Verification items for the finished model (mm, model axes). A direction names the side the tool comes from. Give positions to 0.01 mm unless a question says otherwise; leave off trailing zeros. Loops run counter-clockwise (first coordinate to the right, second up) from the corner with the lowest first, then second, coordinate; pieces in that order, holes last. Notation, with made-up numbers: (18.25, -14.75) - (77.25, -14.75) arc R20 cw to (77.25, 16.25) - close; hole circle Ø3 at (-12, 40). An arc over 180 degrees is marked (long way). One line per question, with ' | ' between items. Start each with the question number.
1. Section check B-B, the plane x = 12. Enter the section's corners in (y, z).
2. Section check A-A, the plane y = 19. Enter the section's corners in (x, z).
3. Tool access check on faces 1 (the face through (27, 69.85, -3)), 2 (the face through (22.86, 16, -3)), 3 (the face through (11, 0, -3)), 4 (the face through (28.53, 64.96, -2.25)), 5 (the face through (27, 57.15, -3)). Record the directions out of +Z, -Z, +X, -X, +Y, -Y that give a thin tool (end or side, any length) a straight path to the whole face; none if there is none.
4. Thickness scan on line 1 along Y through (x, z) = (27, -6); line 2 along Z through (x, y) = (27.5, 38.1). Record the ranges inside material, lowest first. Write a range as from..to.
5. Depth check by flat-ended pin: pin 1 Ø2 at (x, z) = (28, -3.5) entering from -Y; pin 2 Ø1.9 at (y, z) = (13.5, -3) entering from +X; pin 3 Ø5 at (x, y) = (27.5, 76) entering from +Z; pin 4 Ø3 at (x, z) = (28.5, -3.5) entering from +Y. Enter the tip coordinate at first touch or a pass-through.
6. Mould release check, pull along Z, two halves, no side actions. Record for faces 6 (the face through (27, 31.75, -3)), 7 (the face through (28.531, 36.414, -3.549)), 8 (the face through (12, 46, 0)): +Z half, -Z half, draft (parallel to the pull), parting line (faces both ways), or undercut.
from build123d import *

# Parameters (mm, degrees)
SKETCH1_W                 = 31.75
SKETCH1_H                 = 6.35
BOSS_EXTRUDE1_DEPTH       = 101.6
CHAMFER1_SIZE             = 31.75
F_8_32_TAPPED_HOLE1_D     = 3.4544
F_8_32_TAPPED_HOLE1_DEPTH = 6.35
F_8_32_TAPPED_HOLE1_TIP   = 1.037806461
SKETCH4_W                 = 8.89
SKETCH4_H                 = 31.75
SKETCH4_H_2               = 12.7
CUT_EXTRUDE1_DEPTH        = 107.634633211


with BuildPart() as part:
    # Sketch1 → Boss-Extrude1 (new body)
    with BuildSketch(Plane(origin=(0, 0, 0), x_dir=(1, 0, 0), z_dir=(0, 1, 0))):
        with Locations((15.875, 3.175)):
            Rectangle(SKETCH1_W, SKETCH1_H)
    extrude(amount=BOSS_EXTRUDE1_DEPTH)

    # Chamfer1
    chamfer1_edges = [part.edges().sort_by_distance(p)[0] for p in [
        (0, 101.6, -3.175),
    ]]
    chamfer(chamfer1_edges, length=CHAMFER1_SIZE - 0.0001)  # a hair under: the kernel refuses the full size

    # #8-32 Tapped Hole1
    with Locations(Plane(origin=(31.75, 0, 0), x_dir=(0, 0, -1), z_dir=(1, 0, 0))):
        with Locations((3.175, 63.5), (3.175, 38.1)):
            Hole(F_8_32_TAPPED_HOLE1_D / 2, depth=F_8_32_TAPPED_HOLE1_DEPTH)
            with Locations((0, 0, -(F_8_32_TAPPED_HOLE1_DEPTH + F_8_32_TAPPED_HOLE1_TIP / 2))):  # 118° drill point
                Cone(0, F_8_32_TAPPED_HOLE1_D / 2, F_8_32_TAPPED_HOLE1_TIP, mode=Mode.SUBTRACT)

    # Sketch4 → Cut-Extrude1 (cut, through all)
    with BuildSketch(Plane.XY):
        with Locations((27.305, 15.875)):
            Rectangle(SKETCH4_W, SKETCH4_H)
        with Locations((27.305, 50.8)):
            Rectangle(SKETCH4_W, SKETCH4_H_2)
        with Locations((27.305, 85.725)):
            Rectangle(SKETCH4_W, SKETCH4_H)
    extrude(amount=-CUT_EXTRUDE1_DEPTH, mode=Mode.SUBTRACT)


solid = part.part
Results list:
1) outline: (0, -6.35) - (81.85, -6.35) - (81.85, 0) - (0, 0) - close
2) outline: (0, -6.35) - (22.86, -6.35) - (22.86, 0) - (0, 0) - close
3) face 1: +Z, -Z, +X, +Y | face 2: +Z, -Z, +X, -Y | face 3: +Z, -Z, +X, -X, -Y | face 4: +X | face 5: +Z, -Z, +X
4) line 1: 31.75..44.45, 57.15..69.85 | line 2: -6.35..-4.9, -1.45..0
5) pin 1: y = 31.75 | pin 2: x = 22.86 | pin 3: through | pin 4: y = 69.85
6) face 6: draft | face 7: undercut | face 8: +Z half
